Job drawing, mm, ordinate dimensions from the low corner. One solid piece. A direction names the side the tool comes from. Round coordinates to 2 decimals unless told otherwise and drop trailing zeros. Order: outer loops, then holes, each group sorted by start corner. A loop starts at its lowest first (then second) coordinate and runs counter-clockwise, first axis right, second up. Notation, with made-up numbers: (69, 39) -> (122, 39) arc R9 cw to (122, 56) -> close; hole circle Ø3 at (-6, 45.5). An arc over 180 degrees is marked (long way). Return JSON: item names as keys, results as strings. Group by question number.
Q1. Flat gauge pins, fed straight in: pin 1 (10 mm diameter, centred on x = 9.5, y = 64, fed in from +Z); pin 2 (1.5 mm diameter, centred on x = 31.5, z = 23.5, fed in from -Y); pin 3 (1 mm diameter, centred on y = 309.5, z = 30.5, fed in from -X). Where does each tip first touch, or does it go through?
Q2. Cut at C-C (x = 30). Write the cut outline in (y, z), then the cut area to 3 significant figures.
Q3. Probe line 1 along Z through (x, y) = (22, 390); line 2 along Y through (x, z) = (53.5, 24.5); line 3 along X through (y, z) = (122.5, 33). List the from-to ranges inside material, lowest first.
Q4. Which spindle directions (+Z, -Z, +X, -X, +Y, -Y) get a long thin tool onto all of the face, cutting with end or side? Do the marked faces 1 and 2. Say none if no direction does.
Q5. Cut at A-A (y = 367). Write the cut outline in (x, z).
Q6. Cut at B-B (x = 56). Write the cut outline in (y, z), then the cut area to 3 significant figures.
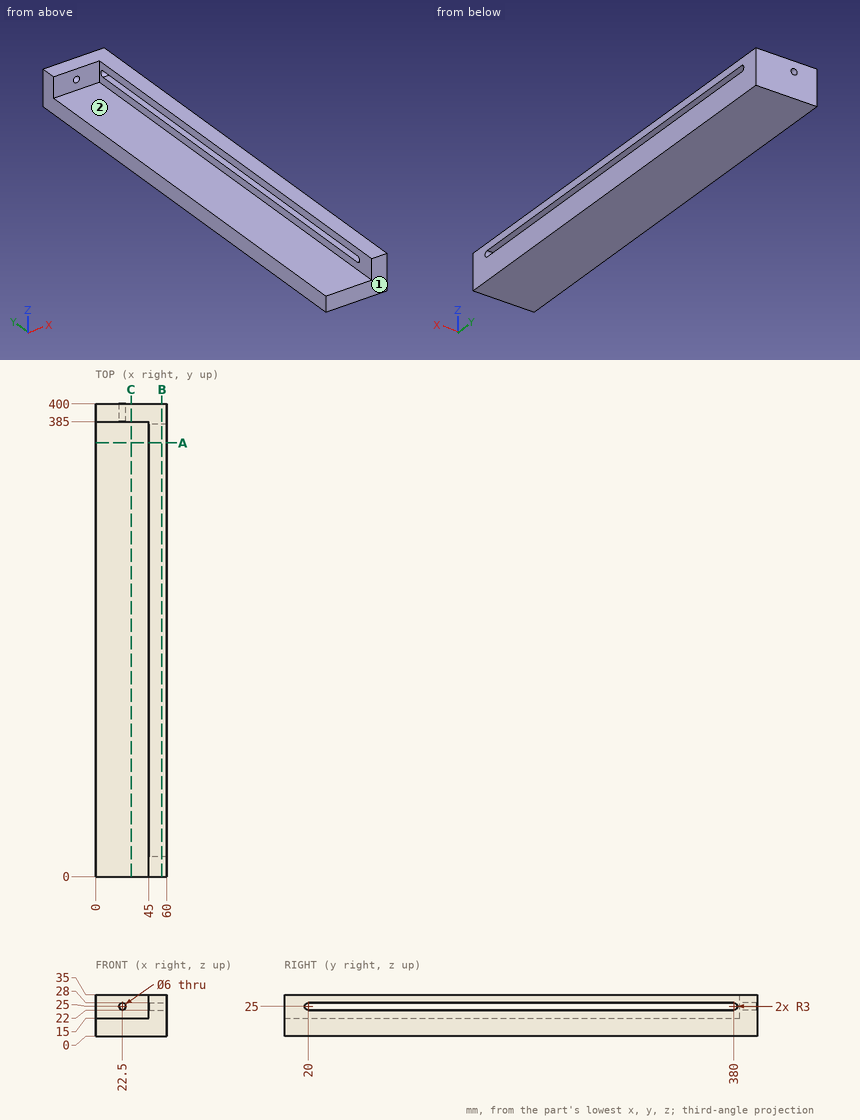
Solution:
{
 "1": {"pin 1": "stops at z = 15", "pin 2": "stops at y = 385", "pin 3": "stops at x = 45"},
 "2": {"outline": "(0, 0) -> (400, 0) -> (400, 35) -> (385, 35) -> (385, 15) -> (0, 15) -> close", "area": "6,300 mm²"},
 "3": {"line 1": "z = 0 to 22.04, 27.96 to 35", "line 2": "y = 0 to 17.04, 382.96 to 400", "line 3": "x = 45 to 60"},
 "4": {"face 1": "+Z, -Z, +X, -X, -Y", "face 2": "+Z, -X, -Y"},
 "5": {"outline": "(0, 0) -> (60, 0) -> (60, 22) -> (45, 22) -> (45, 15) -> (0, 15) -> close; (45, 28) -> (60, 28) -> (60, 35) -> (45, 35) -> close"},
 "6": {"outline": "(0, 0) -> (400, 0) -> (400, 35) -> (0, 35) -> close; hole (20, 22) -> (380, 22) arc R3 ccw to (380, 28) -> (20, 28) arc R3 ccw to start", "area": "11,800 mm²"}
}
